from build123d import *

# Parameters (mm, degrees)
BOSS_EXTRUDE1_DEPTH = 10
SKETCH2_R           = 1.35
CUT_EXTRUDE2_DEPTH  = 56.789784011
FILLET4_R           = 1.5
SKETCH4_W           = 38
SKETCH4_H           = 13
CUT_EXTRUDE3_DEPTH  = 56.789784011
SKETCH5_W           = 50
SKETCH5_H           = 30
CUT_EXTRUDE5_DEPTH  = 2


with BuildPart() as part:
    # Sketch1 → Boss-Extrude1 (new body)
    with BuildSketch(Plane(origin=(0, 0, 0), x_dir=(1, 0, 0), z_dir=(0, 1, 0))):
        with BuildLine():
            Line((-42.5, -27.5), (42.5, -27.5))
            ThreePointArc((42.5, -27.5), (46.035533906, -26.035533906), (47.5, -22.5))
            Line((47.5, -22.5), (47.5, 22.5))
            ThreePointArc((47.5, 22.5), (46.035533906, 26.035533906), (42.5, 27.5))
            Line((42.5, 27.5), (-42.5, 27.5))
            ThreePointArc((-42.5, 27.5), (-46.035533906, 26.035533906), (-47.5, 22.5))
            Line((-47.5, 22.5), (-47.5, -22.5))
            ThreePointArc((-47.5, -22.5), (-46.035533906, -26.035533906), (-42.5, -27.5))
        make_face()
    extrude(amount=BOSS_EXTRUDE1_DEPTH)

    # Sketch2 → Cut-Extrude2 (cut, through all)
    with BuildSketch(Plane(origin=(0, 10, 0), x_dir=(1, 0, 0), z_dir=(0, 1, 0))):
        with Locations(Location((-40, 20, 0), (0, 0, 270))):
            Circle(SKETCH2_R)
        with Locations(Location((-40, -20, 0), (0, 0, 90))):
            Circle(SKETCH2_R)
        with Locations(Location((40, -20, 0), (0, 0, 270))):
            Circle(SKETCH2_R)
        with Locations(Location((40, 20, 0), (0, 0, 90))):
            Circle(SKETCH2_R)
    extrude(amount=-CUT_EXTRUDE2_DEPTH, mode=Mode.SUBTRACT)

    # Fillet4
    fillet4_edges = [part.edges().sort_by_distance(p)[0] for p in [
        (47.5, 0, 0),
        (46.035533906, 0, 26.035533906),
        (0, 0, 27.5),
        (-46.035533906, 0, 26.035533906),
        (-47.5, 0, 0),
        (-46.035533906, 0, -26.035533906),
        (0, 0, -27.5),
        (46.035533906, 0, -26.035533906),
    ]]
    fillet(fillet4_edges, radius=FILLET4_R)

    # Sketch4 → Cut-Extrude3 (cut, through all)
    with BuildSketch(Plane(origin=(0, 0, 0), x_dir=(-1, 0, 0), z_dir=(0, -1, 0))):
        Rectangle(SKETCH4_W, SKETCH4_H)
        with BuildLine():
            Line((20.903728907, -0.502566941), (20.903728907, 0.502566941))
            Line((20.903728907, 0.502566941), (21.927536061, 0.502566941))
            ThreePointArc((21.927536061, 0.502566941), (31.1, 0), (21.927536061, -0.502566941))
            Line((21.927536061, -0.502566941), (20.903728907, -0.502566941))
        make_face()
        with BuildLine():
            Line((-20.903728907, -0.502566941), (-21.927536061, -0.502566941))
            ThreePointArc((-21.927536061, -0.502566941), (-31.1, 0), (-21.927536061, 0.502566941))
            Line((-21.927536061, 0.502566941), (-20.903728907, 0.502566941))
            Line((-20.903728907, 0.502566941), (-20.903728907, -0.502566941))
        make_face()
    extrude(amount=-CUT_EXTRUDE3_DEPTH, mode=Mode.SUBTRACT)

    # Sketch5 → Cut-Extrude5 (cut)
    with BuildSketch(Plane(origin=(0, 10, 0), x_dir=(1, 0, 0), z_dir=(0, 1, 0))):
        Rectangle(SKETCH5_W, SKETCH5_H)
    extrude(amount=-CUT_EXTRUDE5_DEPTH, mode=Mode.SUBTRACT)


solid = part.part
Build history of the part. All positions in model axes, mm. A direction names the side the tool comes from. Coordinates: 2 decimals unless noted, no trailing zeros. Order: outer loops, then holes, each group sorted by start corner. A loop starts at its lowest first (then second) coordinate and runs counter-clockwise, first axis right, second up. Notation, with made-up numbers: (11.25, 79) - (69.25, 79) arc R12 cw to (69.25, 102) - close; hole circle Ø9 at (67, 45.5). An arc over 180 degrees is marked (long way). Put each result on its own line as item: value.
1. Tool access for faces 1 (the face through (25, 9, -10)), 2 (the face through (19, 4, 0)), 3 (the face through (47.5, 6, 0)): list every direction of +Z, -Z, +X, -X, +Y, -Y with a clear straight run to the whole face (end or side of a thin tool).
Answer sheet:
face 1: +Y
face 2: +Y, -Y
face 3: +Z, -Z, +X, +Y, -Y
2. Saw through at D-D (z = 9). Write the cut outline in (x, y), and give its area (3 significant figures).
Answer sheet:
outline: (-47.5, 1.5) arc R1.5 ccw to (-46, 0) - (46, 0) arc R1.5 ccw to (47.5, 1.5) - (47.5, 10) - (25, 10) - (25, 8) - (-25, 8) - (-25, 10) - (-47.5, 10) - close
area: 849 mm^2
3. Probe line 1 along X through (y, z) = (5, 20); line 2 along X through (y, z) = (5.75, 0); line 3 along Z through (x, y) = (1.5, 6.75). List the from-to ranges inside material, lowest first. Write a range as [from, to].
Answer sheet:
line 1: x = [-47.5, -41.35], [-38.65, 38.65], [41.35, 47.5]
line 2: x = [-47.5, -31.1], [-20.9, -19], [19, 20.9], [31.1, 47.5]
line 3: z = [-27.5, -6.5], [6.5, 27.5]
4. Saw through at B-B (y = 6). Write the cut outline in (x, z), and give its area (3 significant figures).
Answer sheet:
outline: (-47.5, -22.5) arc R5 ccw to (-42.5, -27.5) - (42.5, -27.5) arc R5 ccw to (47.5, -22.5) - (47.5, 22.5) arc R5 ccw to (42.5, 27.5) - (-42.5, 27.5) arc R5 ccw to (-47.5, 22.5) - close; hole circle Ø2.7 at (-40, -20); hole circle Ø2.7 at (-40, 20); hole (-21.93, -0.5) - (-20.9, -0.5) - (-20.9, 0.5) - (-21.93, 0.5) arc R4.6 ccw (long way) to start; hole (-19, -6.5) - (19, -6.5) - (19, 6.5) - (-19, 6.5) - close; hole (20.9, -0.5) - (21.93, -0.5) arc R4.6 ccw (long way) to (21.93, 0.5) - (20.9, 0.5) - close; hole circle Ø2.7 at (40, -20); hole circle Ø2.7 at (40, 20)
area: 4,550 mm^2
5. Drop a flat-ended pin along its axis: P1, Ø4, axis at x = -21.5, z = -7.5, coming from the +Y side. Give the stop position or say it passes through.
Answer sheet:
P1: stops at y = 8
6. Saw through at C-C (x = 26.5). Write the cut outline in (y, z), and give its area (3 significant figures).
Answer sheet:
outline: (0, -26) arc R1.5 ccw to (1.5, -27.5) - (10, -27.5) - (10, -4.6) - (0, -4.6) - close; (0, 4.6) - (10, 4.6) - (10, 27.5) - (1.5, 27.5) arc R1.5 ccw to (0, 26) - close
area: 457 mm^2
7. Pull direction Z, two halves, no side cores. Call faces 4 (the face through (46, 5.69, 26.07)), 5 (the face through (-46, 5.69, -26.07)), 6 (the face through (-25, 9, 10)): pulls with the +Z half, pulls with the -Z half, needs draft (parallel to the pull), parting line crosses it, or undercut.
Answer sheet:
face 4: pulls with the +Z half
face 5: pulls with the -Z half
face 6: undercut
8. Saw through at A-A (x = -40). Write the cut outline in (y, z).
Answer sheet:
outline: (0, -26) arc R1.5 ccw to (1.5, -27.5) - (10, -27.5) - (10, -21.35) - (0, -21.35) - close; (0, -18.65) - (10, -18.65) - (10, 18.65) - (0, 18.65) - close; (0, 21.35) - (10, 21.35) - (10, 27.5) - (1.5, 27.5) arc R1.5 ccw to (0, 26) - close
